Autodesk Inventor part; units mm, degrees
ref_plane "YZ Plane" through (0, 0, 0) normal (1, 0, 0) x (0, 1, 0)
ref_plane "XZ Plane" through (0, 0, 0) normal (0, 1, 0) x (-1, 0, 0)
ref_plane "XY Plane" through (0, 0, 0) normal (0, 0, 1) x (1, 0, 0)
sketch "Sketch1" plane through (0, 0, 0) normal (0, 0, 1) x (1, 0, 0)
  line L0 (-53, 50) -> (103, 50)
  line L1 (-53, 50) -> (-53, -100)
  line L2 (-53, -100) -> (103, -100)
  line L3 (103, -100) -> (103, 50)
  line L4 (0, 0) -> (-53, 0)
  line L5 (0, 0) -> (25, 50)
  line L6 (103, 50) -> (23, 50)
  line L7 (-20, -20) -> (20, -20)
  line L8 (20, -20) -> (20, 20)
  line L9 (20, 20) -> (-20, 20)
  line L10 (-20, 20) -> (-20, -20)
  line L11 (-20, -20) -> (20, 20) construction
  line L12 (20, -20) -> (-20, 20) construction
  dimension "d0" = 156
  dimension "d1" = 150
sketch "Sketch2" plane through (0, 0, 0) normal (0, 0, 1) x (1, 0, 0)
  point P0 (0, 0)
extrude "Extrusion1" add sketch "Sketch1" along normal blind 3
sketch "Sketch3" plane through (103, -100, 0) normal (1, 0, 0) x (0, 0, -1)
  point P0 (0, 100)
sketch "Sketch4" plane through (0, 0, 0) normal (0, 0, 1) x (1, 0, 0)
  point P0 (0, 0)
extrude "Extrusion3" cut sketch "Sketch1" along normal blind 10 contours L10 L9 L5 L4 | L4 L5 L9 L8 L7 L10
properties part number "box bottom"
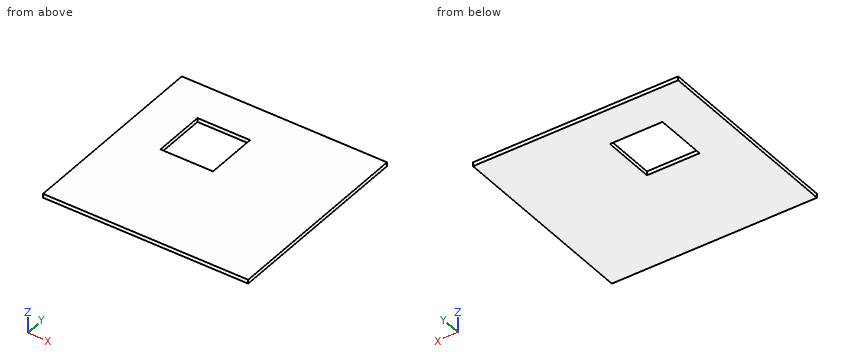
Can you work these out from the model? Positions are in its coordinate system, mm. Round coordinates to 2 decimals unless told otherwise and drop trailing zeros. Order: outer loops, then holes, each group sorted by start corner. A loop starts at its lowest first (then second) coordinate and runs counter-clockwise, first axis right, second up. Notation, with made-up numbers: (82, 63) -> (89, 63) arc R15 ccw to (89, 79) -> close; hole circle Ø3 at (66.25, 72.25). An arc over 180 degrees is marked (long way). Write each question's results on one line, items separated by ' | '. Start each with the question number.
Item 1: If we section it at A-A, the plane y = -8.5: Write out the boundary of the cut face in (x, z), then the cut area to 3 significant figures.
Item 2: Please list where these lines run through material, in increasing order: L1, parallel to X at y = -4, z = 2.5; L2, parallel to Y at x = -18.5, z = 1.45.
Item 3: If we section it at B-B, the plane x = 13: Write out the boundary of the cut face in (y, z), then the cut area to 3 significant figures.
Item 4: If we section it at C-C, the plane z = 0.55: Write out the boundary of the cut face in (x, y).
Results:
1) outline: (-53, 0) -> (-20, 0) -> (-20, 3) -> (-53, 3) -> close; (20, 0) -> (103, 0) -> (103, 3) -> (20, 3) -> close | area: 348 mm2
2) L1: x = -53 to -20, 20 to 103 | L2: y = -100 to -20, 20 to 50
3) outline: (-100, 0) -> (-20, 0) -> (-20, 3) -> (-100, 3) -> close; (20, 0) -> (50, 0) -> (50, 3) -> (20, 3) -> close | area: 330 mm2
4) outline: (-53, -100) -> (103, -100) -> (103, 50) -> (-53, 50) -> close; hole (-20, -20) -> (20, -20) -> (20, 20) -> (-20, 20) -> close
